from build123d import *

# Parameters (mm, degrees)
SKETCH1_W                    = 161.729977966
SKETCH1_H                    = 27.354597718
BASE_FLANGE1_DEPTH           = 0.4826
EDGE_FLANGE1_STRIP_W         = 3.4036
EDGE_FLANGE1_STRIP_H         = 0.4826
EDGE_FLANGE1_STRIP_CUT_DEPTH = 27.354597718
EDGE_FLANGE1_DEPTH           = 27.354597718
EDGE_FLANGE2_STRIP_W         = 3.4036
EDGE_FLANGE2_STRIP_H         = 0.4826
EDGE_FLANGE2_STRIP_CUT_DEPTH = 27.354597718
EDGE_FLANGE2_DEPTH           = 27.354597718
SKETCH12_R                   = 1.27
CUT_EXTRUDE1_DEPTH           = 169.393793797


# Sheet-metal steps are written as plain solids
with BuildPart() as part:
    # Sketch1 → Base-Flange1 (new body)
    with BuildSketch(Plane.XY):
        with Locations((80.864988983, 13.677298859)):
            Rectangle(SKETCH1_W, SKETCH1_H)
    extrude(amount=-BASE_FLANGE1_DEPTH)

    # Edge-Flange1 strip (across the edge) → Edge-Flange1 strip cut (cut)
    with BuildSketch(Plane(origin=(161.729977966, 27.354597718, -0.4826), x_dir=(-1, 0, 0), z_dir=(0, -1, 0))):
        with Locations((-0.4826, -0.2413)):
            Rectangle(EDGE_FLANGE1_STRIP_W, EDGE_FLANGE1_STRIP_H)
    extrude(amount=EDGE_FLANGE1_STRIP_CUT_DEPTH, mode=Mode.SUBTRACT)

    # Edge-Flange1 section (across the edge) → Edge-Flange1 (add)
    with BuildSketch(Plane(origin=(161.729977966, 27.354597718, -0.4826), x_dir=(-1, 0, 0), z_dir=(0, -1, 0))):
        with BuildLine():
            Line((0, 0.7366), (0, 37.6174))
            Line((0, 37.6174), (0.4826, 37.6174))
            Line((0.4826, 37.6174), (0.4826, 0.7366))
            ThreePointArc((0.4826, 0.7366), (0.698345145, 0.215745145), (1.2192, 0))
            Line((1.2192, 0), (1.2192, -0.4826))
            ThreePointArc((1.2192, -0.4826), (0.357095412, -0.125504588), (0, 0.7366))
        make_face()
    extrude(amount=EDGE_FLANGE1_DEPTH)

    # Edge-Flange2 strip (across the edge) → Edge-Flange2 strip cut (cut)
    with BuildSketch(Plane(origin=(0, 0, -0.4826), x_dir=(1, 0, 0), z_dir=(0, 1, 0))):
        with Locations((-0.4826, -0.2413)):
            Rectangle(EDGE_FLANGE2_STRIP_W, EDGE_FLANGE2_STRIP_H)
    extrude(amount=EDGE_FLANGE2_STRIP_CUT_DEPTH, mode=Mode.SUBTRACT)

    # Edge-Flange2 section (across the edge) → Edge-Flange2 (add)
    with BuildSketch(Plane(origin=(0, 0, -0.4826), x_dir=(1, 0, 0), z_dir=(0, 1, 0))):
        with BuildLine():
            Line((0, 0.7366), (0, 37.6174))
            Line((0, 37.6174), (0.4826, 37.6174))
            Line((0.4826, 37.6174), (0.4826, 0.7366))
            ThreePointArc((0.4826, 0.7366), (0.698345145, 0.215745145), (1.2192, 0))
            Line((1.2192, 0), (1.2192, -0.4826))
            ThreePointArc((1.2192, -0.4826), (0.357095412, -0.125504588), (0, 0.7366))
        make_face()
    extrude(amount=EDGE_FLANGE2_DEPTH)

    # Sketch12 → Cut-Extrude1 (cut, through all)
    with BuildSketch(Plane(origin=(161.729977966, 0, 0), x_dir=(0, 0, -1), z_dir=(1, 0, 0))):
        with Locations((21.59, 17.194597718)):
            Circle(SKETCH12_R)
        with Locations((21.59, 9.574597718)):
            Circle(SKETCH12_R)
    extrude(amount=-CUT_EXTRUDE1_DEPTH, mode=Mode.SUBTRACT)


solid = part.part
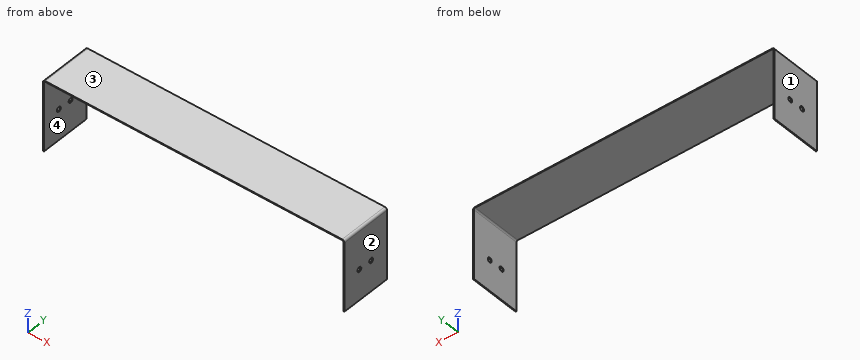
Geometry check sheet. Reference: the model listing, model coordinates, mm. Face numbers are marked on the shaded views. Round coordinates to 2 decimals unless told otherwise and drop trailing zeros. Order: outer loops, then holes, each group sorted by start corner. A loop starts at its lowest first (then second) coordinate and runs counter-clockwise, first axis right, second up. Notation, with made-up numbers: M -8,28 L 2,28 A28 cw 2,64 Z; hole C -4,-33 d9. An arc over 180 degrees is marked long. Answer in a Markdown table with one row per item. Add a question column.
Item 1: Sectioned sample at A-A, the plane z = -15. Enter the section's corners in (x, y), plus the area to 3 significant figures.
Item 2: Draft check along X on the marked faces 1, 2, 3 and 4. Enter one of: released by +X, released by -X, zero draft, split by the parting line, or undercut.
Item 3: Material ranges on L1, parallel to X at y = 13.5, z = -15; L2, parallel to Z at x = 135.5, y = 25.5, recorded low to high. Write a range as [from, to].
Item 4: Sectioned sample at B-B, the plane y = 25. Enter the section's corners in (x, z), plus the area to 3 significant figures.
Item 5: Sectioned sample at C-C, the plane x = 128. Enter the section's corners in (y, z).
Filled in:
| question | item | result |
|---|---|---|
| 1 | outline | M 0,0 L 0.48,0 L 0.48,27.35 L 0,27.35 Z; M 161.25,0 L 161.73,0 L 161.73,27.35 L 161.25,27.35 Z |
| 1 | area | 26.4 mm² |
| 2 | face 1 | released by -X |
| 2 | face 2 | released by +X |
| 2 | face 3 | zero draft |
| 2 | face 4 | undercut |
| 3 | L1 | x = [0, 0.48], [161.25, 161.73] |
| 3 | L2 | z = [-0.48, 0] |
| 4 | outline | M 0,-38.1 L 0.48,-38.1 L 0.48,-1.22 A0.74 cw 1.22,-0.48 L 160.51,-0.48 A0.74 cw 161.25,-1.22 L 161.25,-38.1 L 161.73,-38.1 L 161.73,-1.22 A1.22 ccw 160.51,0 L 1.22,0 A1.22 ccw 0,-1.22 Z |
| 4 | area | 114 mm² |
| 5 | outline | M 0,-0.48 L 27.35,-0.48 L 27.35,0 L 0,0 Z |
